Autodesk Fusion 360 part; units mm, degrees
sketch "extrusion" plane through (0, 0, 0) normal (0, 1, 0) x (1, 0, 0)
  line L0 (-82.5, -8) -> (-62.5, -8)
  line L1 (-62.5, -8) -> (-62.5, 0)
  line L2 (-62.5, 0) -> (62.5, 0)
  line L3 (62.5, 0) -> (62.5, -8)
  line L4 (62.5, -8) -> (82.5, -8)
  line L5 (-60.5, -12) -> (-60.5, -2)
  line L6 (-60.5, -2) -> (60.5, -2)
  line L7 (60.5, -2) -> (60.5, -12)
  line L8 (-82.5, -12) -> (-60.5, -12)
  line L9 (60.5, -12) -> (82.5, -12)
  line L10 (-82.5, -8) -> (-82.5, -12)
  line L11 (82.5, -8) -> (82.5, -12)
  dimension "d1" = 125
  dimension "d2" = 8
  dimension "d3" = 20
  dimension "d4" = 8
  dimension "d5" = 20
extrude "Extrude1" add sketch "extrusion" along normal mid plane 140
sketch "top holes" plane through (0, 0, 12) normal (0, 0, 1) x (-1, 0, 0)
  circle A0 centre (71.5, -53.75) radius 3
  line L0 (82.5, -70) -> (60.5, -70)
  point P0 (71.5, -70)
  dimension "d11" = 6
  dimension "d12" = 16.25
extrude "Extrude2" cut sketch "top holes" against normal blind 4
mirror "Mirror1" about plane through (0, 0, 0) normal (1, 0, 0) of "Extrude2"
mirror "Mirror2" about plane through (0, 0, 0) normal (0, 1, 0) of "Extrude2", "Mirror1"
sketch "Sketch5" plane through (0, 0, 8) normal (0, 0, -1) x (1, 0, 0)
  circle A0 centre (71.5, 53.75) radius 3
  circle A1 centre (71.5, -53.75) radius 3
  line L0 (62.5, 70) -> (62.5, -70)
  line L1 (62.5, -70) -> (82.5, -70)
  line L2 (82.5, -70) -> (82.5, 70)
  line L3 (82.5, 70) -> (62.5, 70)
  circle A2 centre (71.5, 53.75) radius 5
  dimension "d35" = 10
extrude "Extrude6" cut sketch "Sketch5" against normal blind 2 contours A2
sketch "Sketch6" plane through (0, 0, 8) normal (0, 0, -1) x (1, 0, 0)
  circle A0 centre (71.5, 53.75) radius 5
  circle A1 centre (71.5, -53.75) radius 3
  line L0 (62.5, 70) -> (62.5, -70)
  line L1 (62.5, -70) -> (82.5, -70)
  line L2 (82.5, -70) -> (82.5, 70)
  line L3 (82.5, 70) -> (62.5, 70)
  circle A2 centre (71.5, -53.75) radius 5
  dimension "d38" = 10
extrude "Extrude7" cut sketch "Sketch6" against normal blind 2 contours A2
sketch "Sketch7" plane through (0, 0, 8) normal (0, 0, -1) x (1, 0, 0)
  circle A0 centre (-71.5, 53.75) radius 3
  circle A1 centre (-71.5, -53.75) radius 3
  line L0 (-82.5, 70) -> (-82.5, -70)
  line L1 (-82.5, -70) -> (-62.5, -70)
  line L2 (-62.5, -70) -> (-62.5, 70)
  line L3 (-62.5, 70) -> (-82.5, 70)
  circle A2 centre (-71.5, 53.75) radius 5
  dimension "d41" = 10
extrude "Extrude8" cut sketch "Sketch7" against normal blind 2 contours A2
sketch "Sketch8" plane through (0, 0, 8) normal (0, 0, -1) x (1, 0, 0)
  circle A0 centre (-71.5, 53.75) radius 5
  circle A1 centre (-71.5, -53.75) radius 3
  line L0 (-82.5, 70) -> (-82.5, -70)
  line L1 (-82.5, -70) -> (-62.5, -70)
  line L2 (-62.5, -70) -> (-62.5, 70)
  line L3 (-62.5, 70) -> (-82.5, 70)
  circle A2 centre (-71.5, -53.75) radius 5
  dimension "d44" = 10
extrude "Extrude9" cut sketch "Sketch8" against normal blind 2 contours A2
Can you work these out from the model? Positions are in its coordinate system, mm. A direction names the side the tool comes from. Coordinates: 2 decimals unless noted, no trailing zeros. Write each loop counter-clockwise with the first axis right and the second up, starting at its lowest first coordinate (ties: lowest second). Pieces come first, ordered by that corner, then holes. Notation, with made-up numbers: M 79.25,25.5 L 112.25,25.5 A15 ccw 112.25,36.5 Z; hole C 13.5,41.5 d8. An arc over 180 degrees is marked long. Answer as CSV lines item,"result".
Item 1: Imagine slicing it at A-A on x = -71.5. List the corners of the cut face in (y, z) for me.
Geometry results:
outline,"M -70,8 L -58.75,8 L -58.75,10 L -56.75,10 L -56.75,12 L -70,12 Z; M -50.75,10 L -48.75,10 L -48.75,8 L 48.75,8 L 48.75,10 L 50.75,10 L 50.75,12 L -50.75,12 Z; M 56.75,10 L 58.75,10 L 58.75,8 L 70,8 L 70,12 L 56.75,12 Z"
Item 2: Please list where these lines run through material, in increasing order: line 1 along Y through (x, z) = (71.5, 10.55); line 2 along X through (y, z) = (-53.75, 10.95); line 3 along X through (y, z) = (53.75, 9.2).
Geometry results:
line 1,"y = -70 to -56.75, -50.75 to 50.75, 56.75 to 70"
line 2,"x = -82.5 to -74.5, -68.5 to -60.5, 60.5 to 68.5, 74.5 to 82.5"
line 3,"x = -82.5 to -76.5, -66.5 to -60.5, 60.5 to 66.5, 76.5 to 82.5"
Item 3: On a 3-axis mill with a long thin cutter (end or side, diameter ignored), from which of +Z, -Z, +X, -X, +Y, -Y can I reach the whole of each face in a straight line? I mean faces 1 (the flat face through (-73, -1, 8)), 2 (the flat face through (-68, -54, 10)), 3 (the flat face through (72, -1, 8)), 4 (the flat face through (60.5, -1, 7)). Say none if no direction works.
Geometry results:
face 1,"-Z, -X, +Y, -Y"
face 2,"-Z"
face 3,"-Z, +X, +Y, -Y"
face 4,"+Z, +Y, -Y"
Item 4: Imagine slicing it at B-B on y = -53.75. List the corners of the cut face in (x, z) for me, plus the area to 3 significant figures.
Geometry results:
outline,"M -82.5,8 L -76.5,8 L -76.5,10 L -74.5,10 L -74.5,12 L -82.5,12 Z; M -68.5,10 L -66.5,10 L -66.5,8 L -62.5,8 L -62.5,0 L 62.5,0 L 62.5,8 L 66.5,8 L 66.5,10 L 68.5,10 L 68.5,12 L 60.5,12 L 60.5,2 L -60.5,2 L -60.5,12 L -68.5,12 Z; M 74.5,10 L 76.5,10 L 76.5,8 L 82.5,8 L 82.5,12 L 74.5,12 Z"
area,"386 mm2"
Item 5: I'm going to push flat-ended pins straight in: P1, Ø8, axis at x = 74, y = -53.5, coming from the -Z side; P2, Ø8, axis at x = 71.5, y = -53.75, coming from the -Z side; P3, Ø2, axis at x = -19.5, z = 4.5, coming from the -Y side; P4, Ø13, axis at x = 71.5, y = 53.75, coming from the +Z side. Where does each tip first touch, or does it pass through?
Geometry results:
P1,"stops at z = 8"
P2,"stops at z = 10"
P3,"passes through"
P4,"stops at z = 12"
Item 6: Imagine slicing it at C-C on y = 20. List the corners of the cut face in (x, z) for me, plus the area to 3 significant figures.
Geometry results:
outline,"M -82.5,8 L -62.5,8 L -62.5,0 L 62.5,0 L 62.5,8 L 82.5,8 L 82.5,12 L 60.5,12 L 60.5,2 L -60.5,2 L -60.5,12 L -82.5,12 Z"
area,"450 mm2"
Item 7: We'd pull the mould along X, two halves only. Please class faces 5 (the cylindrical face through (-69.29, 51.72, 11.01)), 6 (the flat face through (-72, -1, 12)), 7 (the flat face through (-62.5, -1, 4)): +X half, -X half, draft (parallel to the pull), parting line (faces both ways), or undercut.
Geometry results:
face 5,"undercut"
face 6,"draft"
face 7,"-X half"
